The listing builds one solid part. Answer for the finished solid, in the listing's coordinates (mm). A direction names the side the tool comes from. Give positions to 0.01 mm unless a question says otherwise; leave off trailing zeros. Write each loop counter-clockwise with the first axis right and the second up, starting at its lowest first coordinate (ties: lowest second). Pieces come first, ordered by that corner, then holes.
```python
from build123d import *

# Parameters (mm, degrees)
EXTRUDE1_DEPTH = 20
FILLET1_R      = 1
SKETCH2_R      = 2.55
EXTRUDE2_DEPTH = 24.003477998


with BuildPart() as part:
    # Sketch1 → Extrude1 (new body)
    with BuildSketch(Plane.XY):
        Polygon((0, 0), (8, 0), (8, 1), (10, 1), (10, 2.5), (7.1, 5.4), (0.9, 5.4), (-2, 2.5), (-2, 1), (0, 1), align=None)
    extrude(amount=EXTRUDE1_DEPTH)

    # Fillet1
    fillet1_edges = [part.edges().sort_by_distance(p)[0] for p in [
        (-2, 2.5, 10),
        (0.9, 5.4, 10),
        (7.1, 5.4, 10),
        (10, 2.5, 10),
    ]]
    fillet(fillet1_edges, radius=FILLET1_R)

    # Sketch2 → Extrude2 (cut, through all)
    with BuildSketch(Plane(origin=(0, 5.4, 0), x_dir=(1, 0, 0), z_dir=(0, 1, 0))):
        with Locations(Location((4, -10, 0), (0, 0, 270))):
            Circle(SKETCH2_R)
    extrude(amount=-EXTRUDE2_DEPTH, mode=Mode.SUBTRACT)


solid = part.part
```
Item 1: A cutting plane is placed at D-D, the plane y = 3.8. Give the vertices of the cut face in (x, z), plus the area to 3 significant figures.
Conclusion:
outline: (-0.7, 0) - (8.7, 0) - (8.7, 20) - (-0.7, 20) - close; hole circle Ø5.1 at (4, 10)
area: 168 mm2
Item 2: A cutting plane is placed at B-B, the plane z = 10. Give the vertices of the cut face in (x, y), plus the area to 3 significant figures.
Conclusion:
outline: (-2, 1) - (0, 1) - (0, 0) - (1.45, 0) - (1.45, 5.4) - (1.31, 5.4) arc R1 ccw to (0.61, 5.11) - (-1.71, 2.79) arc R1 ccw to (-2, 2.09) - close; (6.55, 0) - (8, 0) - (8, 1) - (10, 1) - (10, 2.09) arc R1 ccw to (9.71, 2.79) - (7.39, 5.11) arc R1 ccw to (6.69, 5.4) - (6.55, 5.4) - close
area: 24.8 mm2
Item 3: A cutting plane is placed at A-A, the plane x = 4. Give the vertices of the cut face in (y, z).
Conclusion:
outline: (0, 0) - (5.4, 0) - (5.4, 7.45) - (0, 7.45) - close; (0, 12.55) - (5.4, 12.55) - (5.4, 20) - (0, 20) - close
Item 4: Which of the six approach directions +Z, -Z, +X, -X, +Y, -Y give full straight-line access (tool end or side, diameter ignored) to faces 4 (the face through (0, 0.5, 9.9)), 5 (the face through (8, 0.5, 9.9)), 6 (the face through (-0.5, 4, 9.9))?
Conclusion:
face 4: +Z, -Z, -X, -Y
face 5: +Z, -Z, +X, -Y
face 6: +Z, -Z, -X, +Y
Item 5: Consider probe 1 along X at (y, z) = (1.8, 10); probe 2 along Y at (x, z) = (1.25, 3); probe 3 along Z at (x, y) = (5.75, 0.6). Determine where each line is inside the solid, lowest interval first.
Conclusion:
probe 1: x = -2 to 1.45, 6.55 to 10
probe 2: y = 0 to 5.4
probe 3: z = 0 to 8.15, 11.85 to 20
Item 6: Determine the mould class of faces 1 (the face through (4, 3, 0)), 2 (the face through (6.15, 2.74, 11.37)), 3 (the face through (10, 1.5, 9.9)) for opening direction Z: pulls with the +Z half, pulls with the -Z half, needs draft (parallel to the pull), parting line crosses it, or undercut.
Conclusion:
face 1: pulls with the -Z half
face 2: undercut
face 3: needs draft
Item 7: A cutting plane is placed at C-C, the plane z = 17.75. Give the vertices of the cut face in (x, y).
Conclusion:
outline: (-2, 1) - (0, 1) - (0, 0) - (8, 0) - (8, 1) - (10, 1) - (10, 2.09) arc R1 ccw to (9.71, 2.79) - (7.39, 5.11) arc R1 ccw to (6.69, 5.4) - (1.31, 5.4) arc R1 ccw to (0.61, 5.11) - (-1.71, 2.79) arc R1 ccw to (-2, 2.09) - close
